Model file for the job. Use its own axes, mm. Face numbers are marked on the shaded views. A direction names the side the tool comes from. Coordinates: 2 decimals unless noted, no trailing zeros. Write each loop counter-clockwise with the first axis right and the second up, starting at its lowest first coordinate (ties: lowest second). Pieces come first, ordered by that corner, then holes. Notation, with made-up numbers: M 47,15 L 60,15 A11 ccw 60,29 Z; hole C 60.5,0 d2. An arc over 180 degrees is marked long. One line per question, with ' | ' between items. Start each with the question number.
(1) Wall check: probe 1 along Z at (x, y) = (42, 481); probe 2 along Y at (x, z) = (268, 120.5); probe 3 along Y at (x, z) = (433.5, 61). Give the ranges that are in metal, low to high.
(2) Flat gauge pins, fed straight in: pin 1 Ø1 at (y, z) = (658, 111) entering from +X; pin 2 Ø4 at (x, y) = (506, 543) entering from +Z; pin 3 Ø4 at (x, z) = (509.5, 99) entering from +Y. Where does each tip first touch, or does it go through?
(3) Cut at B-B (x = 478). Write the cut outline in (y, z), plus the area to 3 significant figures.
(4) Cut at C-C (y = 698). Write the cut outline in (x, z), plus the area to 3 significant figures.
(5) Cut at D-D (z = 184.5). Write the cut outline in (x, y), plus the area to 3 significant figures.
(6) Cut at A-A (z = 64). Write the cut outline in (x, y).
(7) Tool access for the marked faces 1 and 2: list every direction of +Z, -Z, +X, -X, +Y, -Y with a clear straight run to the whole face (end or side of a thin tool).
from build123d import *

# Parameters (mm, degrees)
BOSS_EXTRUDE1_DEPTH = 101.6
BOSS_EXTRUDE2_DEPTH = 576.302521
CUT_EXTRUDE1_DEPTH  = 132.021743181
CUT_EXTRUDE2_DEPTH  = 132.021743181


with BuildPart() as part:
    # Sketch1 → Boss-Extrude1 (new body)
    with BuildSketch(Plane.XY):
        Polygon((0, 0), (576.302521008, 0), (576.302521008, 387.403361345), (502.663865546, 560.294117647), (355.386554622, 762), (198.504201681, 762), (102.453781513, 637.134453782), (0, 448.235294118), align=None)
    extrude(amount=BOSS_EXTRUDE1_DEPTH)

    # Sketch2 → Boss-Extrude2 (add)
    with BuildSketch(Plane.ZY):
        Polygon((101.6, 0), (232.621743181, 0), (232.621743181, 198.64821401), (204.451845393, 430.506603568), (172.780455352, 570.81191653), (155.089264466, 615.704741573), (155.089264466, 670.908278379), (139.607943989, 752.787376516), (101.6, 762), align=None)
    extrude(amount=-BOSS_EXTRUDE2_DEPTH)

    # Sketch3 → Cut-Extrude1 (cut, through all)
    with BuildSketch(Plane(origin=(0, 0, 101.6), x_dir=(-1, 0, 0), z_dir=(0, 0, -1))):
        Polygon((0, 448.235294118), (-102.079559314, 636.444481603), (-205.052343037, 770.512583763), (-205.052343037, 987.342816442), (227.879484492, 941.92173413), (179.71587047, 482.849418415), align=None)
    extrude(amount=-CUT_EXTRUDE1_DEPTH, mode=Mode.SUBTRACT)

    # Sketch4 → Cut-Extrude2 (cut, through all)
    with BuildSketch(Plane(origin=(0, 0, 101.6), x_dir=(-1, 0, 0), z_dir=(0, 0, -1))):
        Polygon((-576.302521008, 387.403361345), (-502.663865546, 560.294117647), (-355.386554622, 762), (-386.647779508, 961.526140846), (-935.090979015, 961.526140846), (-884.913915701, 472.949119069), align=None)
    extrude(amount=-CUT_EXTRUDE2_DEPTH, mode=Mode.SUBTRACT)


solid = part.part
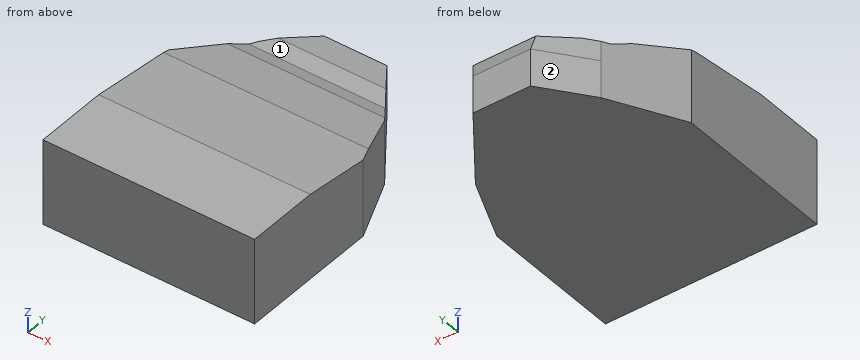
Filled in:
1) probe 1: 0 to 193.05 | probe 2: 0 to 757.42 | probe 3: 0 to 655.02
2) pin 1: x = 431.69 | pin 2: z = 179.51 | pin 3: y = 548.94
3) outline: M 0,0 L 594.07,0 L 594.07,163.61 L 570.81,172.78 L 430.51,204.45 L 198.65,232.62 L 0,232.62 Z | area: 127,000 mm²
4) outline: M 149.27,0 L 402.12,0 L 402.12,149.97 L 149.36,149.97 L 149.36,101.6 L 149.27,101.6 Z | area: 37,900 mm²
5) outline: M 0,0 L 576.3,0 L 576.3,387.4 L 520.3,518.89 L 38.32,518.89 L 0,448.24 Z | area: 294,000 mm²
6) outline: M 0,0 L 576.3,0 L 576.3,387.4 L 502.66,560.29 L 355.39,762 L 198.5,762 L 102.45,637.13 L 0,448.24 Z
7) face 1: +Z, +X, -X, +Y | face 2: +Z, -Z, -X, +Y
